Part model, mm, in its own coordinate system. A direction names the side the tool comes from. Round coordinates to 2 decimals unless told otherwise and drop trailing zeros. Write each loop counter-clockwise with the first axis right and the second up, starting at its lowest first coordinate (ties: lowest second). Pieces come first, ordered by that corner, then holes. Notation, with made-up numbers: (-38, 1) -> (-21, 1) arc R16 cw to (-21, 14) -> close; hole circle Ø6 at (51.25, -27.75). An arc over 180 degrees is marked (long way). Return JSON: item names as keys, results as strings. Group by question number.
(1) Saw through at D-D (y = 99). List the corners of the cut face in (x, z), plus the area to 3 significant figures.
(2) Saw through at C-C (x = 37). List the corners of the cut face in (y, z).
(3) Drill centre lines: L1, parallel to Z at x = -28, y = -39; L2, parallel to X at y = 75.5, z = 2.45; L3, parallel to Y at x = 4.5, z = 0.35. Where is each one in solid material? Low to high. Write a range as from..to.
(4) Tool access for faces 1 (the flat face through (47.31, -59.65, 1.4)), 2 (the flat face through (-1, 1, 0)): list every direction of +Z, -Z, +X, -X, +Y, -Y with a clear straight run to the whole face (end or side of a thin tool).
(5) Saw through at A-A (y = -29.5). List the corners of the cut face in (x, z), plus the area to 3 significant figures.
from build123d import *

# Parameters (mm, degrees)
F0_W     = 109.6518
F0_H     = 149.225
F1_DEPTH = 2.8448
F3_DEPTH = 25.4
F5_DEPTH = 3.048
F9_DEPTH = 107.442


# Not quite as in the source:
# - a feature names something its author has since deleted; it is built from what else it names


with BuildPart() as f1:
    # F0 (on Top) → F1 (new body)
    with BuildSketch(Plane.XY):
        with Locations((13.2645608256, 0)):
            Rectangle(F0_W, F0_H)
    extrude(amount=F1_DEPTH)

    # F2 (on face) → F3 (cut)
    with BuildSketch(Plane.XY.offset(2.8448)):
        Polygon((68.0904608256, -74.6125), (27.7860667557, -74.6125), (68.0904608256, -75.2405971289), align=None)
        Polygon((-41.5613391744, -75.712069869), (-25.0190570951, -74.6125), (-41.5613391744, -74.6125), align=None)
    extrude(amount=-F3_DEPTH, mode=Mode.SUBTRACT)

    # F4 (on face) → F5 (join)
    with BuildSketch(Plane.XY.offset(2.8448)):
        with BuildLine():
            Line((-41.5613391744, 74.6125), (68.0904608256, 74.6125))
            ThreePointArc((68.0904608256, 74.6125), (13.2645608256, 129.4384), (-41.5613391744, 74.6125))
        make_face()
    extrude(amount=-F5_DEPTH)


with BuildPart() as f1_1:
    # F6: moved
    add(f1.part.moved(Location((-10.668, 0, 0))))


with BuildPart() as f1_2:
    # F7: moved
    add(f1_1.part.moved(Location((-2.794, 0, 0))))

    # F8 (on Top) → F9 (cut)
    with BuildSketch(Plane.XY):
        Polygon((-55.1044642925, -45.067888195), (-55.1044642925, -74.785888195), (-40.1565642925, -74.785888195), align=None)
        Polygon((54.6766667015, -45.0012958965), (39.7287667015, -74.7192958965), (54.6766667015, -74.7192958965), align=None)
    extrude(amount=F9_DEPTH, mode=Mode.SUBTRACT)


solid = f1_2.part
Computed values:
{
 "1": {"outline": "(-49.3, -0.2) -> (48.91, -0.2) -> (48.91, 2.84) -> (-49.3, 2.84) -> close", "area": "299 mm2"},
 "2": {"outline": "(-74.61, 0) -> (74.61, 0) -> (74.61, -0.2) -> (114.89, -0.2) -> (114.89, 2.84) -> (-74.61, 2.84) -> close"},
 "3": {"L1": "0..2.84", "L2": "-55.02..54.62", "L3": "-74.61..129.24"},
 "4": {"face 1": "+Z, -Z, +X, -Y", "face 2": "-Z, +X, -X, -Y"},
 "5": {"outline": "(-55.02, 0) -> (54.63, 0) -> (54.63, 2.84) -> (-55.02, 2.84) -> close", "area": "312 mm2"}
}
